Geometry check sheet. Reference: the model listing, model coordinates, mm. Face numbers are marked on the shaded views. Give positions to 0.01 mm unless a question says otherwise; leave off trailing zeros. Loops run counter-clockwise (first coordinate to the right, second up) from the corner with the lowest first, then second, coordinate; pieces in that order, holes last. Notation, with made-up numbers: (87, 57.5) -> (126, 57.5) arc R24 ccw to (126, 94.5) -> close; hole circle Ø6 at (32, 60). An arc over 180 degrees is marked (long way). One line per question, with ' | ' between items.
from build123d import *

# Parameters (mm, degrees)
CROQUIS1_R              = 20
CROQUIS1_R_2            = 3
SALIENTE_EXTRUIR1_DEPTH = 5


with BuildPart() as part:
    # Croquis1 → Saliente-Extruir1 (new body)
    with BuildSketch(Plane.XY):
        Circle(CROQUIS1_R)
        with Locations((10, 0)):
            Circle(CROQUIS1_R_2, mode=Mode.SUBTRACT)
        with Locations((-10, 0)):
            Circle(CROQUIS1_R_2, mode=Mode.SUBTRACT)
        with BuildLine():
            ThreePointArc((8.75, 4.841229183), (0, 10), (-8.75, 4.841229183))
            ThreePointArc((-8.75, 4.841229183), (-5, 0), (-8.75, -4.841229183))
            ThreePointArc((-8.75, -4.841229183), (0, -10), (8.75, -4.841229183))
            ThreePointArc((8.75, -4.841229183), (5, 0), (8.75, 4.841229183))
        make_face(mode=Mode.SUBTRACT)
    extrude(amount=SALIENTE_EXTRUIR1_DEPTH)


solid = part.part
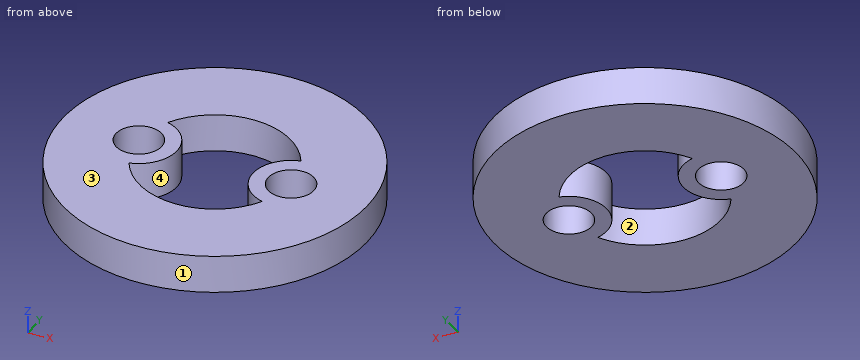
Item 1: Sectioned sample at D-D (y = -12). Record the cut outline in (x, z).
Result:
outline: (-16, 0) -> (16, 0) -> (16, 5) -> (-16, 5) -> close
Item 2: Sectioned sample at A-A (y = 0). Record the cut outline in (x, z), plus the area to 3 significant figures.
Result:
outline: (-20, 0) -> (-13, 0) -> (-13, 5) -> (-20, 5) -> close; (-7, 0) -> (-5, 0) -> (-5, 5) -> (-7, 5) -> close; (5, 0) -> (7, 0) -> (7, 5) -> (5, 5) -> close; (13, 0) -> (20, 0) -> (20, 5) -> (13, 5) -> close | area: 90.0 mm2
Item 3: Scan lines: probe 1 along X at (y, z) = (-0.5, 1.35); probe 2 along X at (y, z) = (7, 1.7) (3 decimals); probe 3 along Y at (x, z) = (-0.5, 1.7). Record each from-to range of solid material in increasing order.
Result:
probe 1: -19.99 to -12.96, -7.04 to -5.03, 5.03 to 7.04, 12.96 to 19.99 | probe 2: -18.735 to -7.141, 7.141 to 18.735 | probe 3: -19.99 to -9.99, 9.99 to 19.99
Item 4: Release check for a two-part mould opening along Y. For the marked faces 1, 2, 3 and 4 record: pulls with the +Y half, pulls with the -Y half, needs draft (parallel to the pull), parting line crosses it, or undercut.
Result:
face 1: parting line crosses it | face 2: undercut | face 3: needs draft | face 4: undercut
Item 5: Depth check by flat-ended pin: pin 1 Ø3 at (x, z) = (13.5, 3) entering from +Y; pin 2 Ø3.5 at (x, y) = (10, 0) entering from -Z; pin 3 Ø1 at (x, z) = (2.5, 3) entering from +Y. Enter the tip coordinate at first touch or a pass-through.
Result:
pin 1: y = 16 | pin 2: through | pin 3: y = 19.9
Item 6: Sectioned sample at C-C (x = -2). Record the cut outline in (y, z), plus the area to 3 significant figures.
Result:
outline: (-19.9, 0) -> (-9.8, 0) -> (-9.8, 5) -> (-19.9, 5) -> close; (9.8, 0) -> (19.9, 0) -> (19.9, 5) -> (9.8, 5) -> close | area: 101 mm2
Item 7: Sectioned sample at B-B (z = 0.75). Record the cut outline in (x, y).
Result:
outline: circle Ø40 at (0, 0); hole circle Ø6 at (-10, 0); hole (-8.75, -4.84) arc R10 ccw to (8.75, -4.84) arc R5 cw to (8.75, 4.84) arc R10 ccw to (-8.75, 4.84) arc R5 cw to start; hole circle Ø6 at (10, 0)
